Here's how the part is built. I have some questions about the finished solid (model axes, mm). Face numbers are marked on the shaded views. Round coordinates to 2 decimals unless told otherwise and drop trailing zeros. Write each loop counter-clockwise with the first axis right and the second up, starting at its lowest first coordinate (ties: lowest second). Pieces come first, ordered by that corner, then holes. Notation, with made-up numbers: (88, -24) -> (145, -24) arc R22 ccw to (145, 5) -> close; hole circle Ø10 at (25, 22.25). An arc over 180 degrees is marked (long way). Answer in a Markdown table with one row per item.
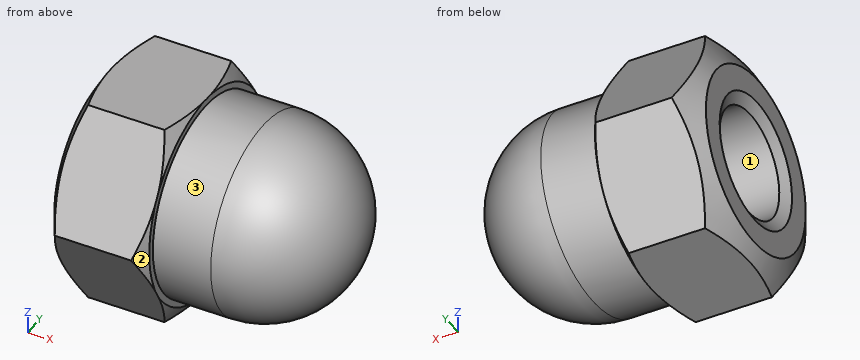
Autodesk Inventor part; units mm, degrees
ref_plane "Work Plane1" through (3.6771, 0, 0) normal (0, 0.866, -0.5) x (-1, 0, 0)
ref_plane "YZ Plane" through (0, 0, 0) normal (1, 0, 0) x (0, 1, 0)
ref_plane "XZ Plane" through (0, 0, 0) normal (0, 1, 0) x (-1, 0, 0)
sketch "Sketch1" plane through (0, 0, 0) normal (1, 0, 0) x (0, 1, 0)
  line L0 (-2.3094, -4) -> (-4.6188, 0)
  line L1 (-4.6188, 0) -> (-2.3094, 4)
  line L2 (-2.3094, 4) -> (2.3094, 4)
  line L3 (2.3094, 4) -> (4.6188, 0)
  line L4 (4.6188, 0) -> (2.3094, -4)
  line L5 (2.3094, -4) -> (-2.3094, -4)
  point P0 (0, 0)
  point P1 (0, 0)
  dimension "d0" = 9.2376
extrude "Body" add sketch "Sketch1" along normal blind 4
sketch "Sketch2" plane through (0, 0, 0) normal (0, 0, 1) x (1, 0, 0)
  line L0 (4, 0) -> (10, 0)
  arc A0 (10, 0) -> (6.25, 3.75) centre (6.25, 0) ccw
  line L1 (6.25, 3.75) -> (4, 3.75)
  line L2 (4, -2.3094) -> (4, 2.3094)
  line L3 (4, 0) -> (4, 3.75)
  line L4 (2.6447, 0) -> (12.132, 0)
  dimension "d8" = 3.75
  dimension "d9" = 6
revolve "Cap" add sketch "Sketch2" angle 360 about axis through (4, 0, 0) along (1, 0, 0)
sketch "Sketch3" plane through (0, 0, 0) normal (-1, 0, 0) x (0, 0, 1)
  line L0 (0, -6.4663) -> (0, 6.4663)
  line L1 (-5.6, 0) -> (5.6, 0)
  point P0 (0, 0)
hole "Thread" at (0, 0, 0) direction (1, 0, 0) diameter 4.134 depth 7.3542 tip angle 120
sketch "Sketch4" plane through (0, 0, 0) normal (0, 0, 1) x (1, 0, 0)
  line L0 (0, 2.3094) -> (0, 4.6188)
  line L1 (0, 4.6188) -> (4, 4.6188)
  line L2 (4, 2.3094) -> (4, 4.6188)
  line L3 (-0.8, 0) -> (4.8, 0)
  line L4 (0.6748, 4.6188) -> (0, 3.45)
  line L5 (3.6427, 4.6188) -> (4, 4)
  dimension "d3" = 6.9
  dimension "d4" = 30
  dimension "d5" = 8
  dimension "d6" = 30
revolve "Chamfer1" cut sketch "Sketch4" angle 360 about axis through (-10, 0, 0) along (1, 0, 0)
chamfer "Chamfer2" distance 0.433 angle 30 1 edges at (0, 0, -2.067) measured on face at (0, 2.9506, -0.3583)
ref_plane "Work Plane1" through (3.6771, 0, 0) normal (0, 0.866, -0.5) x (-1, 0, 0)
equation "\"d0\" = 1.1547 * SW"
equation "\"d1\" = SIH"
equation "\"d8\" = KR"
equation "\"d9\" = KOH1 - SIH"
equation "\"d11\" = GEL"
equation "\"d12\" = 1.02 * GEL"
equation "\"d3\" = SW0"
equation "\"d4\" = ANG1"
equation "\"d5\" = SW01"
equation "\"d6\" = ANG2"
equation "\"d14\" = -0.5 * GD1 + 0.5 * NND"
equation "\"d36\" = -0.5 * GD1 + 0.5 * NND"
equation "\"ANG1\" = 30deg"
equation "\"ANG2\" = 30deg"
equation "\"NND\" = 5"
equation "\"SIH\" = 4"
equation "\"KOH1\" = 10"
equation "\"GEL\" = 7.21"
equation "\"SW\" = 8"
equation "\"KR\" = 3.75"
equation "\"SW0\" = 6.9"
equation "\"SW01\" = SW"
equation "\"GUL\" = 0.541266 * PTC"
equation "\"THREADDIA\" = 5"
equation "\"TOA\" = 30deg"
equation "\"PTC\" = 0.8"
equation "\"E0\" = 1.155 * SW"
equation "\"GAL\" = 0.541266 * PTC"
properties part number "DIN 1587 - M5" material "Steel, Mild"
1) I want a section at A-A, the plane x = 3.25. List the corners of the cut face in (y, z) for me, and give its area (3 significant figures).
Response:
| item | result |
|---|---|
| outline | (-4.62, 0) -> (-2.31, -4) -> (2.31, -4) -> (4.62, 0) -> (2.31, 4) -> (-2.31, 4) -> close; hole circle Ø4.13 at (0, 0) |
| area | 42.0 mm^2 |
2) I need wall thicknesses on line 1 (Z direction, x = 3.25, y = 0); line 2 (Z direction, x = 5.5, y = 0); line 3 (X direction, y = -0.75, z = 1.25). Which ranges of each line are inside material? Lowest first, please. Write a range as [from, to].
Response:
| item | result |
|---|---|
| line 1 | z = [-4, -2.07], [2.07, 4] |
| line 2 | z = [-3.75, -2.07], [2.07, 3.75] |
| line 3 | x = [7.71, 9.71] |
3) I want a section at B-B, the plane x = 4.75. List the corners of the cut face in (y, z) for me, and give its area (3 significant figures).
Response:
| item | result |
|---|---|
| outline | circle Ø7.5 at (0, 0); hole circle Ø4.13 at (0, 0) |
| area | 30.8 mm^2 |
4) For pin 1 (1 mm diameter, centred on x = 3.5, y = -3.5, fed in from -Z); pin 2 (2 mm diameter, centred on x = 2, z = 2.5, fed in from -Y); pin 3 (2.5 mm diameter, centred on y = 1.5, z = 0, fed in from +X), each with a flat end and sliding along its axis, tell me the tip position at first contact or that it passes through.
Response:
| item | result |
|---|---|
| pin 1 | stops at z = -2.8 |
| pin 2 | stops at y = -3.75 |
| pin 3 | stops at x = 9.99 |
5) We'd pull the mould along Y, two halves only. Please class the marked faces 1, 2 and 3: +Y half, -Y half, draft (parallel to the pull), parting line (faces both ways), or undercut.
Response:
| item | result |
|---|---|
| face 1 | undercut |
| face 2 | -Y half |
| face 3 | parting line |
